Can you work these out from the model? Positions are in its coordinate system, mm. A direction names the side the tool comes from. Give positions to 0.01 mm unless a question says otherwise; leave off trailing zeros. Loops run counter-clockwise (first coordinate to the right, second up) from the corner with the lowest first, then second, coordinate; pieces in that order, holes last.
from build123d import *

# Parameters (mm, degrees)
F0_W     = 110
F0_H     = 40
F1_DEPTH = 65
F2_R     = 5.5
F3_DEPTH = 80
F2_R_2   = 9
F4_DEPTH = 57.3
F5_R     = 14
F6_DEPTH = 80


with BuildPart() as f1:
    # F0 (on Top) → F1 (new body)
    with BuildSketch(Plane.XY):
        Rectangle(F0_W, F0_H)
    extrude(amount=F1_DEPTH)

    # F2 (on face) → F3 (cut)
    with BuildSketch(Plane.XY.offset(65)):
        with Locations((-40, 0)):
            Circle(F2_R)
        with Locations((40, 0)):
            Circle(F2_R)
    extrude(amount=-F3_DEPTH, mode=Mode.SUBTRACT)

    # F2 (on face) → F4 (cut)
    with BuildSketch(Plane.XY.offset(65)):
        with Locations((-40, 0)):
            Circle(F2_R_2)
        with Locations((-40, 0)):
            Circle(F2_R, mode=Mode.SUBTRACT)
        with Locations((40, 0)):
            Circle(F2_R_2)
        with Locations((40, 0)):
            Circle(F2_R, mode=Mode.SUBTRACT)
    extrude(amount=-F4_DEPTH, mode=Mode.SUBTRACT)

    # F5 (on face) → F6 (cut)
    with BuildSketch(Plane.XZ.offset(20)):
        with Locations((0, 40)):
            Circle(F5_R)
        with BuildLine():
            Line((-55, 65), (-55, 15))
            Line((-55, 15), (-25, 15))
            Line((-25, 15), (-25, 40))
            ThreePointArc((-25, 40), (-17.67767, 57.67767), (0, 65))
            Line((0, 65), (-55, 65))
        make_face()
        with BuildLine():
            Line((55, 65), (0, 65))
            ThreePointArc((0, 65), (17.67767, 57.67767), (25, 40))
            Line((25, 40), (25, 15))
            Line((25, 15), (55, 15))
            Line((55, 15), (55, 65))
        make_face()
    extrude(amount=-F6_DEPTH, mode=Mode.SUBTRACT)


solid = f1.part
(1) Suppose I cut it at B-B on x = -40. List the corners of the cut face in (y, z) for me.
Returned:
outline: (-20, 0) - (-5.5, 0) - (-5.5, 7.7) - (-9, 7.7) - (-9, 15) - (-20, 15) - close; (5.5, 0) - (20, 0) - (20, 15) - (9, 15) - (9, 7.7) - (5.5, 7.7) - close
(2) Suppose I cut it at C-C on y = -11.5. List the corners of the cut face in (x, z) for me.
Returned:
outline: (-55, 0) - (55, 0) - (55, 15) - (25, 15) - (25, 40) arc R25 ccw to (0, 65) arc R25 ccw to (-25, 40) - (-25, 15) - (-55, 15) - close; hole circle Ø28 at (0, 40)
(3) Suppose I cut it at D-D on z = 44.5. List the corners of the cut face in (x, y) for me.
Returned:
outline: (-24.59, -20) - (-13.26, -20) - (-13.26, 20) - (-24.59, 20) - close; (13.26, -20) - (24.59, -20) - (24.59, 20) - (13.26, 20) - close
(4) Thinking about a two-plate mould opening in X: for faces 4 (the flat face through (-25, 0, 27)), 5 (the flat face through (-40.2, -9.2, 15)), 6 (the cylindrical face through (-3.03, -0.28, 26.33)), 7 (the cylindrical face through (31, 0, 11)), which applies, pulls with the +X half, pulls with the -X half, needs draft (parallel to the pull), parting line crosses it, or undercut?
Returned:
face 4: pulls with the -X half
face 5: needs draft
face 6: undercut
face 7: undercut
(5) Please list where these lines run through material, in increasing order: probe 1 along Y at (x, z) = (40, 6); probe 2 along X at (y, z) = (-2.5, 17.5); probe 3 along Z at (x, y) = (0, 9.5).
Returned:
probe 1: y = -20 to -5.5, 5.5 to 20
probe 2: x = -25 to 25
probe 3: z = 0 to 26, 54 to 65
(6) Will these pins go through, and if not, where does the flat tip stop? P1, Ø12, axis at x = 16.5, y = -5, coming from the +Z side; P2, Ø1, axis at y = -3, z = 18.5, coming from the +X side; P3, Ø15, axis at x = 42.5, y = 0, coming from the +Z side; P4, Ø22.5, axis at x = 0, z = 40, coming from the +Y side.
Returned:
P1: stops at z = 62.69
P2: stops at x = 25
P3: stops at z = 15
P4: passes through
(7) Which directions (+Z, -Z, +X, -X, +Y, -Y) give clear straight access to the entire face, cutting with the end or side of a thin tool? Please do faces 1 (the flat face through (39.8, -9.2, 15)), 2 (the flat face through (55, 0, 7)), 3 (the flat face through (-36, 4, 7.7)).
Returned:
face 1: +Z, +X, +Y, -Y
face 2: +Z, -Z, +X, +Y, -Y
face 3: +Z
(8) Suppose I cut it at A-A on y = 0. List the corners of the cut face in (x, z) for me.
Returned:
outline: (-55, 0) - (-45.5, 0) - (-45.5, 7.7) - (-49, 7.7) - (-49, 15) - (-55, 15) - close; (-34.5, 0) - (34.5, 0) - (34.5, 7.7) - (31, 7.7) - (31, 15) - (25, 15) - (25, 40) arc R25 ccw to (0, 65) arc R25 ccw to (-25, 40) - (-25, 15) - (-31, 15) - (-31, 7.7) - (-34.5, 7.7) - close; (45.5, 0) - (55, 0) - (55, 15) - (49, 15) - (49, 7.7) - (45.5, 7.7) - close; hole circle Ø28 at (0, 40)
